from build123d import *

# Parameters (mm, degrees)
PAD_DEPTH       = 2
SKETCH001_R     = 4
SKETCH001_W     = 56
SKETCH001_H     = 15
SKETCH001_H_2   = 10
POCKET_DEPTH    = 2.001
SKETCH002_W     = 70.645367
SKETCH002_H     = 8.666905
POCKET001_DEPTH = 107
FILLET_R        = 2


with BuildPart() as part:
    # Sketch → Pad (new body)
    with BuildSketch(Plane.XY):
        with BuildLine():
            Line((-32, 110), (-32, 0))
            Line((-32, 0), (32, 0))
            Line((32, 0), (32, 110.000041))
            ThreePointArc((32, 110.000041), (-2.1e-05, 142), (-32, 110))
        make_face()
    extrude(amount=PAD_DEPTH)

    # Sketch001 (on DatumPlane) → Pocket (cut, through all)
    with BuildSketch(Plane.XY.offset(2)):
        with Locations((0, 132.667633)):
            Circle(SKETCH001_R)
        with Locations((0, 11.5)):
            Rectangle(SKETCH001_W, SKETCH001_H)
        with Locations((0, 28.5)):
            Rectangle(SKETCH001_W, SKETCH001_H)
        with Locations((0, 45.5)):
            Rectangle(SKETCH001_W, SKETCH001_H)
        with Locations((0, 62.5)):
            Rectangle(SKETCH001_W, SKETCH001_H)
        with Locations((0, 79.5)):
            Rectangle(SKETCH001_W, SKETCH001_H)
        with Locations((0, 97)):
            Rectangle(SKETCH001_W, SKETCH001_H_2)
    extrude(amount=-POCKET_DEPTH, mode=Mode.SUBTRACT)

    # Sketch002 (on DatumPlane) → Pocket001 (cut)
    with BuildSketch(Plane.XZ):
        with Locations((-0.08378, -0.285264)):
            Rectangle(SKETCH002_W, SKETCH002_H)
        Polygon((29.8, 2), (-29.8, 2), (-31.8, 0.6), (-31.8, 0), (31.8, 0), (31.8, 0.6), align=None, mode=Mode.SUBTRACT)
    extrude(amount=-POCKET001_DEPTH, mode=Mode.SUBTRACT)

    # Fillet
    fillet_edges = [part.edges().sort_by_distance(p)[0] for p in [
        (-31.8, 0, 0.3),
        (31.8, 0, 0.3),
    ]]
    fillet(fillet_edges, radius=FILLET_R)


solid = part.part
Input: part model. Units: mm. Frame: model coordinates. Give positions to 0.01 mm unless a question says otherwise; leave off trailing zeros. Order: outer loops, then holes, each group sorted by start corner. A loop starts at its lowest first (then second) coordinate and runs counter-clockwise, first axis right, second up. Notation, with made-up numbers: (47.5, -33.75) -> (74.5, -33.75) arc R9 ccw to (74.5, -24.75) -> close; hole circle Ø3 at (64.5, -12). An arc over 180 degrees is marked (long way). Use one line per item in the form item = value.
1) Section A-A, the plane x = 0. Count the separate pieces of the cut face and the enclosed holes in it, and give its area (3 significant figures).
Response values:
separate_pieces = 8
enclosed_holes = 0
area = 98.0 mm^2
2) Mould query, pull axis X, two halves, no side actions, for faces 1 (the cylindrical face through (0.704, 141.992, 0.986)), 2 (the flat face through (0, 88, 0)), 3 (the cylindrical face through (-0.867, 128.763, 1.014)). Classes: pulls with the +X half, pulls with the -X half, needs draft (parallel to the pull), parting line crosses it, or undercut.
Response values:
face_1 = parting line crosses it
face_2 = needs draft
face_3 = undercut
3) Section B-B, the plane y = 43. Return loops of the section in (x, z).
Response values:
outline = (-31.8, 0) -> (-28, 0) -> (-28, 2) -> (-29.8, 2) -> (-31.8, 0.6) -> close; (28, 0) -> (31.8, 0) -> (31.8, 0.6) -> (29.8, 2) -> (28, 2) -> close
4) First-contact query: pin 1 Ø1 at (x, z) = (-6.5, 0.5) entering from +Y; pin 2 Ø0.6 at (y, z) = (78, 0.5) entering from -X; pin 3 Ø0.6 at (y, z) = (66, 0.5) entering from +X. Flat tips, straight axial feed; report the tip coordinate or a pass-through.
Response values:
pin_1 = 141.43
pin_2 = -31.8
pin_3 = 31.8
5) Line query: probe 1 along X at (y, z) = (31.5, 0.15); probe 2 along X at (y, z) = (26, 1.75); probe 3 along X at (y, z) = (112, 0.3). Output: solid intervals per line, ascending.
Response values:
probe_1 = -31.8 to -28, 28 to 31.8
probe_2 = -30.16 to -28, 28 to 30.16
probe_3 = -31.94 to 31.94
6) Section C-C, the plane x = -23. Return loops of the section in (y, z), and give its area (3 significant figures).
Response values:
outline = (0, 0) -> (4, 0) -> (4, 2) -> (0, 2) -> close; (19, 0) -> (21, 0) -> (21, 2) -> (19, 2) -> close; (36, 0) -> (38, 0) -> (38, 2) -> (36, 2) -> close; (53, 0) -> (55, 0) -> (55, 2) -> (53, 2) -> close; (70, 0) -> (72, 0) -> (72, 2) -> (70, 2) -> close; (87, 0) -> (92, 0) -> (92, 2) -> (87, 2) -> close; (102, 0) -> (132.25, 0) -> (132.25, 2) -> (102, 2) -> close
area = 94.5 mm^2
